```python
from build123d import *

# Parameters (mm, degrees)
CROQUIS1_W              = 67
CROQUIS1_H              = 28
SALIENTE_EXTRUIR1_DEPTH = 7
CROQUIS2_W              = 60.9
CROQUIS2_H              = 21.9
CORTAR_EXTRUIR1_DEPTH   = 4
CORTAR_EXTRUIR5_DEPTH   = 3


with BuildPart() as part:
    # Croquis1 → Saliente-Extruir1 (new body)
    with BuildSketch(Plane.XY):
        with Locations((-40.002156686, 17.680995475)):
            Rectangle(CROQUIS1_W, CROQUIS1_H)
    extrude(amount=SALIENTE_EXTRUIR1_DEPTH)

    # Croquis2 → Cortar-Extruir1 (cut)
    with BuildSketch(Plane.XY.offset(7)):
        with Locations((-40.002156686, 17.680995475)):
            Rectangle(CROQUIS2_W, CROQUIS2_H)
    extrude(amount=-CORTAR_EXTRUIR1_DEPTH, mode=Mode.SUBTRACT)

    # Croquis6 → Cortar-Extruir5 (cut)
    with BuildSketch(Plane(origin=(0, 0, 0), x_dir=(-1, 0, 0), z_dir=(0, 0, -1))):
        with BuildLine():
            Line((46.002156686, 15.680995475), (48.317498248, 15.680995475))
            ThreePointArc((48.317498248, 15.680995475), (61.002156686, 17.680995475), (48.317498248, 19.680995475))
            Line((48.317498248, 19.680995475), (46.002156686, 19.680995475))
            ThreePointArc((46.002156686, 19.680995475), (44.002156686, 17.680995475), (46.002156686, 15.680995475))
        make_face()
    extrude(amount=-CORTAR_EXTRUIR5_DEPTH, mode=Mode.SUBTRACT)


solid = part.part
```
Could you check a few things on this model? Use its own coordinates, in mm. A direction names the side the tool comes from. Give positions to 0.01 mm unless a question says otherwise; leave off trailing zeros. Write each loop counter-clockwise with the first axis right and the second up, starting at its lowest first coordinate (ties: lowest second). Pieces come first, ordered by that corner, then holes. Notation, with made-up numbers: (83, -30.75) -> (114, -30.75) arc R19 ccw to (114, -13.75) -> close; hole circle Ø9 at (2.5, -14). An arc over 180 degrees is marked (long way). Write each question's results on one line, items separated by ' | '.
1. On a 3-axis mill with a long thin cutter (end or side, diameter ignored), from which of +Z, -Z, +X, -X, +Y, -Y can I reach the whole of each face in a straight line? I mean faces 5 (the flat face through (-47, 15.681, 1)), 6 (the flat face through (-40, 18, 0)), 7 (the flat face through (-40, 18, 3)). Say none if no direction works.
Check sheet entries:
face 5: +Z, -Z | face 6: -Z, +X, -X, +Y, -Y | face 7: +Z
2. I want a section at B-B, the plane y = 14.5. Write out the boundary of the cut face in (x, z), then the cut area to 3 significant figures.
Check sheet entries:
outline: (-73.5, 0) -> (-60.17, 0) -> (-60.17, 3) -> (-70.45, 3) -> (-70.45, 7) -> (-73.5, 7) -> close; (-48.83, 0) -> (-6.5, 0) -> (-6.5, 7) -> (-9.55, 7) -> (-9.55, 3) -> (-48.83, 3) -> close | area: 191 mm²
3. If we mould it in two halves opening along Y, with no side actions, what happens to faces 1 (the flat face through (-40, 31.681, 3)), 2 (the flat face through (-47, 19.681, 1)), 3 (the flat face through (-43, 6, 7)), 4 (the flat face through (-40, 6.731, 5))? For each: released by +Y, released by -Y, zero draft, split by the parting line, or undercut.
Check sheet entries:
face 1: released by +Y | face 2: undercut | face 3: zero draft | face 4: undercut
4. I want a section at C-C, the plane x = -65. Write out the boundary of the cut face in (y, z), then the cut area to 3 significant figures.
Check sheet entries:
outline: (3.68, 0) -> (31.68, 0) -> (31.68, 7) -> (28.63, 7) -> (28.63, 3) -> (6.73, 3) -> (6.73, 7) -> (3.68, 7) -> close | area: 108 mm²
5. Will this pin go through, and if not, where does the flat tip stop? pin 1 Ø11 at (x, y) = (-33.5, 21) entering from +Z.
Check sheet entries:
pin 1: stops at z = 3
6. I need wall thicknesses on L1, parallel to X at y = 18, z = 5; L2, parallel to Y at x = -31, z = 6; L3, parallel to Z at x = -34.5, y = 15.25. Which ranges of each line are inside material? Lowest first, please.
Check sheet entries:
L1: x = -73.5 to -70.45, -9.55 to -6.5 | L2: y = 3.68 to 6.73, 28.63 to 31.68 | L3: z = 0 to 3
7. I want a section at A-A, the plane z = 1. Write out the boundary of the cut face in (x, y).
Check sheet entries:
outline: (-73.5, 3.68) -> (-6.5, 3.68) -> (-6.5, 31.68) -> (-73.5, 31.68) -> close; hole (-48.32, 15.68) -> (-46, 15.68) arc R2 ccw to (-46, 19.68) -> (-48.32, 19.68) arc R6.5 ccw (long way) to start
8. I want a section at D-D, the plane y = 9.75. Write out the boundary of the cut face in (x, z).
Check sheet entries:
outline: (-73.5, 0) -> (-6.5, 0) -> (-6.5, 7) -> (-9.55, 7) -> (-9.55, 3) -> (-70.45, 3) -> (-70.45, 7) -> (-73.5, 7) -> close
